```python
from build123d import *

# Parameters (mm, degrees)
F0_W     = 8.5
F0_H     = 24
F0_W_2   = 7
F0_H_2   = 12
F0_W_3   = 5
F1_DEPTH = 2.5
F2_DEPTH = 13.5
F3_R     = 1
F4_DEPTH = 12.5
F5_R     = 5
F6_R     = 5


with BuildPart() as f1:
    # F0 (on Top) → F1 (new body)
    with BuildSketch(Plane.XY):
        with Locations((12.10625, 0.3)):
            Rectangle(F0_W, F0_H)
        Polygon((-3.14375, 35.3), (-7.14375, 35.3), (-7.14375, 15.3), (-7.14375, 12.3), (-7.14375, -11.7), (-7.14375, -14.7), (-7.14375, -34.7), (-3.14375, -34.7), (-3.14375, -22.7), (3.85625, -22.7), (3.85625, -34.7), (7.85625, -34.7), (7.85625, -14.7), (7.85625, -11.7), (7.85625, 12.3), (7.85625, 15.3), (7.85625, 35.3), (3.85625, 35.3), (3.85625, 23.3), (-3.14375, 23.3), align=None)
        with Locations((0.35625, 29.3)):
            Rectangle(F0_W_2, F0_H_2)
        with Locations((0.35625, -28.7)):
            Rectangle(F0_W_2, F0_H_2)
        Polygon((-7.14375, 15.3), (-7.14375, 35.3), (-20.64375, 15.3), align=None)
        Polygon((21.35625, 15.3), (7.85625, 35.3), (7.85625, 15.3), align=None)
        Polygon((-7.14375, -34.7), (-7.14375, -14.7), (-20.64375, -14.7), align=None)
        Polygon((21.35625, -14.7), (7.85625, -14.7), (7.85625, -34.7), align=None)
        with Locations((-18.14375, 0.3)):
            Rectangle(F0_W_3, F0_H)
        with Locations((18.85625, 0.3)):
            Rectangle(F0_W_3, F0_H)
        Polygon((-7.14375, 12.3), (-7.14375, 15.3), (-20.64375, 15.3), (-20.64375, 12.3), (-15.64375, 12.3), align=None)
        Polygon((-7.14375, -14.7), (-7.14375, -11.7), (-15.64375, -11.7), (-20.64375, -11.7), (-20.64375, -14.7), align=None)
        Polygon((21.35625, 15.3), (7.85625, 15.3), (7.85625, 12.3), (16.35625, 12.3), (21.35625, 12.3), align=None)
        Polygon((16.35625, -11.7), (7.85625, -11.7), (7.85625, -14.7), (21.35625, -14.7), (21.35625, -11.7), align=None)
        with Locations((-11.39375, 0.3)):
            Rectangle(F0_W, F0_H)
    extrude(amount=F1_DEPTH)

    # F0 (on Top) → F2 (join)
    with BuildSketch(Plane.XY):
        Polygon((-3.14375, 35.3), (-7.14375, 35.3), (-7.14375, 15.3), (-7.14375, 12.3), (-7.14375, -11.7), (-7.14375, -14.7), (-7.14375, -34.7), (-3.14375, -34.7), (-3.14375, -22.7), (3.85625, -22.7), (3.85625, -34.7), (7.85625, -34.7), (7.85625, -14.7), (7.85625, -11.7), (7.85625, 12.3), (7.85625, 15.3), (7.85625, 35.3), (3.85625, 35.3), (3.85625, 23.3), (-3.14375, 23.3), align=None)
    extrude(amount=F2_DEPTH)

    # F3 (on Right) → F4 (cut, symmetric)
    with BuildSketch(Plane.YZ):
        with Locations((-30, 9.5)):
            Circle(F3_R)
        with Locations((30, 9.5)):
            Circle(F3_R)
    extrude(amount=F4_DEPTH, both=True, mode=Mode.SUBTRACT)

    # F5
    f5_edges = [f1.edges().sort_by_distance(p)[0] for p in [
        (-5.14375, -34.7, 13.5),
        (5.85625, -34.7, 13.5),
    ]]
    fillet(f5_edges, radius=F5_R)

    # F6
    f6_edges = [f1.edges().sort_by_distance(p)[0] for p in [
        (5.85625, 35.3, 13.5),
        (-5.14375, 35.3, 13.5),
    ]]
    fillet(f6_edges, radius=F6_R)


solid = f1.part
```
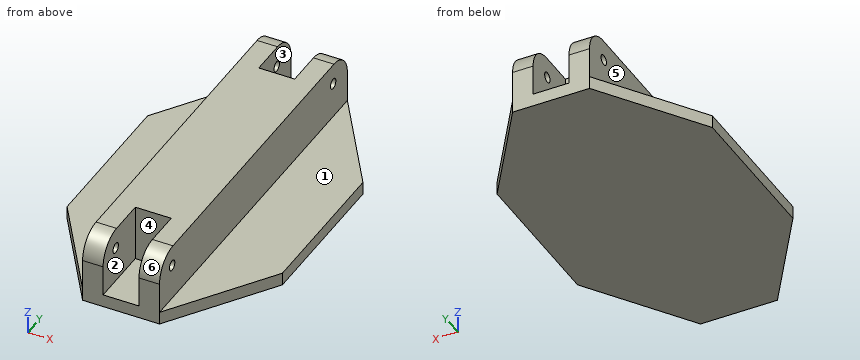
Work out the finished part from the listing and answer in its coordinate system (mm). Face numbers are marked on the shaded views. A direction names the side the tool comes from. Give positions to 0.01 mm unless a question says otherwise; leave off trailing zeros. Loops run counter-clockwise (first coordinate to the right, second up) from the corner with the lowest first, then second, coordinate; pieces in that order, holes last. Notation, with made-up numbers: M -23.75,76.25 L -7.75,76.25 A27 ccw -7.75,100.25 Z; hole C 65.25,38.25 d4. An arc over 180 degrees is marked long. One line per item, written item: value. Start each with the question number.
1. Find section B-B (x = 6). Give the vertices of the cut face in (y, z), and give its area (3 significant figures).
2. Determine the mould class of the marked faces 4, 5 and 6 for opening direction X: released by +X, released by -X, zero draft, split by the parting line, or undercut.
3. Find section D-D (y = -18). Give the vertices of the cut face in (x, z).
4. Which of the six approach directions +Z, -Z, +X, -X, +Y, -Y give full straight-line access (tool end or side, diameter ignored) to the marked faces 1, 2 and 3?
5. Find section A-A (z = 9.5). Give the vertices of the cut face in (x, y).
6. Find section C-C (y = 8). Give the vertices of the cut face in (x, z).
7. Each of these flat-tipped pins is pushed along its axis until it touches: P1, Ø5.5, axis at y = -30, z = 6.5, coming from the +X side; P2, Ø7, axis at x = -16, y = -6, coming from the +Z side; P3, Ø2, axis at x = 1, z = 8, coming from the -Y side. Where does it stop, or does it pass through?
8. Find the intervals of material crossed by probe 1 along X at (y, z) = (31.5, 12.25); probe 2 along Z at (x, y) = (-4.1, -30); probe 3 along X at (y, z) = (9.5, 12), in increasing order.
Reported:
1. outline: M -34.7,0 L 35.3,0 L 35.3,8.5 A5 ccw 30.3,13.5 L -29.7,13.5 A5 ccw -34.7,8.5 Z; hole C -30,9.5 d2; hole C 30,9.5 d2
1. area: 928 mm²
2. face 4: undercut
2. face 5: released by -X
2. face 6: zero draft
3. outline: M -18.42,0 L 19.13,0 L 19.13,2.5 L 7.86,2.5 L 7.86,13.5 L -7.14,13.5 L -7.14,2.5 L -18.42,2.5 Z
4. face 1: +Z, +X, +Y, -Y
4. face 2: +Z, -Y
4. face 3: +Z, +Y
5. outline: M -7.14,-34.6 L -3.14,-34.6 L -3.14,-31 L -7.14,-31 Z; M -7.14,-29 L -3.14,-29 L -3.14,-22.7 L 3.86,-22.7 L 3.86,-29 L 7.86,-29 L 7.86,29 L 3.86,29 L 3.86,23.3 L -3.14,23.3 L -3.14,29 L -7.14,29 Z; M -7.14,31 L -3.14,31 L -3.14,35.2 L -7.14,35.2 Z; M 3.86,-34.6 L 7.86,-34.6 L 7.86,-31 L 3.86,-31 Z; M 3.86,31 L 7.86,31 L 7.86,35.2 L 3.86,35.2 Z
6. outline: M -20.64,0 L 21.36,0 L 21.36,2.5 L 7.86,2.5 L 7.86,13.5 L -7.14,13.5 L -7.14,2.5 L -20.64,2.5 Z
7. P1: stops at x = 7.86
7. P2: stops at z = 2.5
7. P3: stops at y = -22.7
8. probe 1: x = -7.14 to -3.14, 3.86 to 7.86
8. probe 2: z = 0 to 8.5, 10.5 to 13.49
8. probe 3: x = -7.14 to 7.86
